For this review, take the finished solid that the model builds, in its own axes (mm). A direction names the side the tool comes from. Round coordinates to 2 decimals unless told otherwise and drop trailing zeros. Loops run counter-clockwise (first coordinate to the right, second up) from the corner with the lowest first, then second, coordinate; pieces in that order, holes last. Notation, with made-up numbers: (1.25, 35.25) -> (56.25, 35.25) arc R30 ccw to (56.25, 64.25) -> close; hole circle Ø10 at (15, -37.75). An arc over 180 degrees is marked (long way). One line per question, with ' | ' between items. Start each with the question number.
1. Consider section A-A (z = 0). Write out the cut boundary in (x, y) (3 decimals), and give its area (3 significant figures).
2. Consider section D-D (z = 28.5). Write out the cut boundary in (x, y) (3 decimals).
3. For faces 1 (the face through (25, -15.875, -8)), 2 (the face through (-9, -18.415, 17.5)), list the 3-axis set-ups (+Z, -Z, +X, -X, +Y, -Y) from which the entire face can be reached by the end or side of a thin tool; tool diameter is ignored.
4. For pin 1 Ø8 at (y, z) = (-10.5, -20) entering from -X; pin 2 Ø5 at (x, y) = (26, -2.5) entering from +Z; pin 3 Ø1.5 at (y, z) = (-2.5, 13.5) entering from +X; pin 4 Ø1.5 at (y, z) = (-8.5, 13.5) entering from -X, all flat-tipped, find the tip position at first contact; note any pin that passes through.
5. Consider section C-C (y = -4.25). Write out the cut boundary in (x, z).
6. Consider section B-B (x = 0). Write out the cut boundary in (y, z) (3 decimals).
7. Draft analysis for pull direction Z (two halves, no side actions). For faces 3 (the face through (-30.235, -17.163, -23.183)), 4 (the face through (8, 0, -18)), 5 (the face through (-15.319, -9.079, 11.746)), state which applies: pulls with the +Z half, pulls with the -Z half, needs draft (parallel to the pull), parting line crosses it, or undercut.
8. Wall thickness on line 1 along Z through (x, y) = (0, -12.5); line 2 along Y through (x, z) = (-24.5, -25) (3 decimals); line 3 along X through (y, z) = (-14.5, 4.5): over which ranges is each line inside the solid? List them lowest first.
Autodesk Inventor part; units mm, degrees
ref_plane "YZ Plane" through (0, 0, 0) normal (1, 0, 0) x (0, 1, 0)
ref_plane "XZ Plane" through (0, 0, 0) normal (0, 1, 0) x (-1, 0, 0)
ref_plane "XY Plane" through (0, 0, 0) normal (0, 0, 1) x (1, 0, 0)
sketch "Sketch1" plane through (0, 0, 0) normal (0, 0, 1) x (1, 0, 0)
  line L0 (21.844, 0) -> (21.844, -12.7)
  line L1 (25.019, -15.875) -> (38.1, -15.875)
  line L2 (38.1, -15.875) -> (38.1, -18.415)
  line L3 (38.1, -18.415) -> (19.304, -18.415)
  line L4 (19.304, -18.415) -> (19.304, 0)
  line L5 (19.304, 0) -> (21.844, 0)
  line L6 (0, 0) -> (27.9096, 0) construction
  arc A0 (21.844, -12.7) -> (25.019, -15.875) centre (25.019, -12.7) ccw
  line L7 (0, 0) -> (0, -18.415) construction
  dimension "d0" = 19.304
  dimension "d1" = 18.415
  dimension "d2" = 2.54
  dimension "d3" = 2.54
  dimension "d5" = 3.175
  dimension "d9" = 38.1
revolve "Revolution1" add sketch "Sketch1" angle 360 about axis through (0, 0, 0) along (0, -1, 0)
sketch "Sketch2" plane through (0, 0, 0) normal (1, 0, 0) x (0, 1, 0)
  line L0 (0, 0) -> (-26.67, 0) construction
  line L1 (-13.97, -6.35) -> (0, -6.35)
  line L2 (0, -6.35) -> (0, 6.35)
  line L3 (0, 6.35) -> (-13.97, 6.35)
  line L4 (-13.97, 6.35) -> (-13.97, -6.35)
  line L5 (-13.97, -6.35) -> (0, 6.35) construction
  line L6 (0, -6.35) -> (-13.97, 6.35) construction
  line L7 (0, 19.304) -> (0, -19.304)
  point P0 (-6.985, 0)
  dimension "d10" = 12.7
  dimension "d11" = 13.97
  dimension "d12" = 0
properties part number "customWasherTmp"
Answer block:
1) outline: (-38.1, -18.415) -> (-19.304, -18.415) -> (-19.304, 0) -> (-21.844, 0) -> (-21.844, -12.7) arc R3.175 cw to (-25.019, -15.875) -> (-38.1, -15.875) -> close; (19.304, -18.415) -> (38.1, -18.415) -> (38.1, -15.875) -> (25.019, -15.875) arc R3.175 cw to (21.844, -12.7) -> (21.844, 0) -> (19.304, 0) -> close | area: 180 mm2
2) outline: (-25.286, -18.415) -> (25.286, -18.415) -> (25.286, -15.875) -> (-25.286, -15.875) -> close
3) face 1: +Y | face 2: +Z, -Z, +X, -X, -Y
4) pin 1: stops at x = -14.87 | pin 2: passes through | pin 3: stops at x = 17.74 | pin 4: stops at x = -17.74
5) outline: circle Ø43.69 at (0, 0); hole circle Ø38.61 at (0, 0)
6) outline: (-18.415, -38.1) -> (-15.875, -38.1) -> (-15.875, -25.019) arc R3.175 cw to (-12.7, -21.844) -> (0, -21.844) -> (0, -19.304) -> (-18.415, -19.304) -> close; (-18.415, 19.304) -> (0, 19.304) -> (0, 21.844) -> (-12.7, 21.844) arc R3.175 cw to (-15.875, 25.019) -> (-15.875, 38.1) -> (-18.415, 38.1) -> close
7) face 3: parting line crosses it | face 4: needs draft | face 5: undercut
8) line 1: z = -21.84 to -19.3, 19.3 to 21.84 | line 2: y = -18.415 to -15.875 | line 3: x = -21.95 to -18.77, 18.77 to 21.95
